Study the drawing (mm; zero at the part's minimum x, y, z) and answer. A direction names the side the tool comes from. Give positions to 0.01 mm unless a question says otherwise; leave off trailing zeros. Write each loop counter-clockwise with the first axis right and the second up, starting at its lowest first coordinate (ties: lowest second). Pieces come first, ordered by that corner, then holes. Notation, with made-up numbers: (16, 47.25) -> (68, 47.25) arc R13 ccw to (68, 65.25) -> close; hole circle Ø4 at (-35, -29.75). An arc over 180 degrees is marked (long way). One line per question, with ' | ' between items.
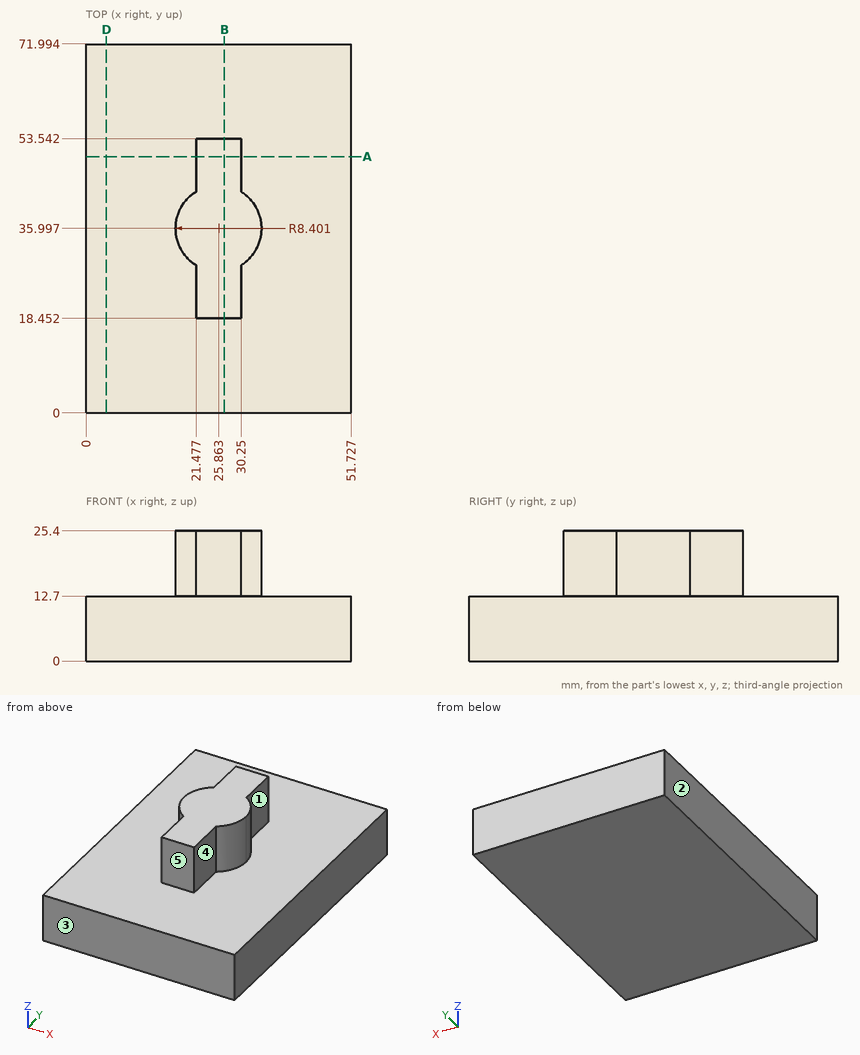
Item 1: A tool of negligible diameter and unlimited length cuts with its end or side. For the marked faces 1, 2, 3, 4 and 5, from which of +Z, -Z, +X, -X, +Y, -Y can it reach the whole face along a straight path? Write none if from no direction.
Answers below:
face 1: +Z, +X, +Y | face 2: +Z, -Z, -X, +Y, -Y | face 3: +Z, -Z, +X, -X, -Y | face 4: +Z, +X, -Y | face 5: +Z, +X, -X, -Y
Item 2: Consider line 1 (Z direction, x = 35.5, y = 18); line 2 (Y direction, x = 27, z = 19.25); line 3 (X direction, y = 20.5, z = 16.5). Determine where each line is inside the solid, lowest interval first. Write a range as [from, to].
Answers below:
line 1: [0, 12.7] | line 2: [18.45, 53.54] | line 3: [21.48, 30.25]
Item 3: Find section D-D (x = 4). Write down the section's boundary in (y, z).
Answers below:
outline: (0, 0) -> (71.99, 0) -> (71.99, 12.7) -> (0, 12.7) -> close
Item 4: Find section A-A (y = 50). Write down the section's boundary in (x, z), then the cut area to 3 significant figures.
Answers below:
outline: (0, 0) -> (51.73, 0) -> (51.73, 12.7) -> (30.25, 12.7) -> (30.25, 25.4) -> (21.48, 25.4) -> (21.48, 12.7) -> (0, 12.7) -> close | area: 768 mm²
Item 5: Find section B-B (x = 27). Write down the section's boundary in (y, z).
Answers below:
outline: (0, 0) -> (71.99, 0) -> (71.99, 12.7) -> (53.54, 12.7) -> (53.54, 25.4) -> (18.45, 25.4) -> (18.45, 12.7) -> (0, 12.7) -> close
Item 6: Flat-ended cylindrical pins translate along their axes: pin 1 (5 mm diameter, centred on x = 6.5, y = 46, fed in from +Z); pin 2 (9.5 mm diameter, centred on x = 26, z = 21.5, fed in from -Y); pin 3 (8.5 mm diameter, centred on y = 24, z = 20, fed in from -X). Find the tip coordinate at first contact, or state that the pin passes through.
Answers below:
pin 1: z = 12.7 | pin 2: y = 18.45 | pin 3: x = 21.48
